from build123d import *

# Parameters (mm, degrees)
F0_W      = 200
F0_H      = 100
F1_DEPTH  = 20
F3_DEPTH  = 10
F5_DEPTH  = 10
F6_R      = 45
F7_DEPTH  = 10
F8_R      = 30
F9_DEPTH  = 32
F11_D     = 10
F11_DEPTH = 15
F11_TIP   = 3.0043030951


with BuildPart() as f1:
    # F0 (on Top) → F1 (new body)
    with BuildSketch(Plane.XY):
        Rectangle(F0_W, F0_H)
    extrude(amount=F1_DEPTH)

    # F2 (on face) → F3 (cut)
    with BuildSketch(Plane.XY.offset(20)):
        with BuildLine():
            Line((-75, 40), (-81, 40))
            ThreePointArc((-81, 40), (-89.4852813742, 36.4852813742), (-93, 28))
            Line((-93, 28), (-93, -28))
            ThreePointArc((-93, -28), (-89.4852813742, -36.4852813742), (-81, -40))
            Line((-81, -40), (-75, -40))
            ThreePointArc((-75, -40), (-66.5147186258, -36.4852813742), (-63, -28))
            Line((-63, -28), (-63, 28))
            ThreePointArc((-63, 28), (-66.5147186258, 36.4852813742), (-75, 40))
        make_face()
    extrude(amount=-F3_DEPTH, mode=Mode.SUBTRACT)

    # F4 (on face) → F5 (join)
    with BuildSketch(Plane.XY.offset(20)):
        with BuildLine():
            Line((45.028, 48), (-43, 48))
            ThreePointArc((-43, 48), (-50.0710678119, 45.0710678119), (-53, 38))
            Line((-53, 38), (-53, -38))
            ThreePointArc((-53, -38), (-50.0710678119, -45.0710678119), (-43, -48))
            Line((-43, -48), (45.028, -48))
            ThreePointArc((45.028, -48), (49.7542524478, -47.0300742427), (53.7164858981, -44.2770896333))
            Line((53.7164858981, -44.2770896333), (86.0406073726, -10.3463620417))
            ThreePointArc((86.0406073726, -10.3463620417), (90.18, 0), (86.0406073726, 10.3463620417))
            Line((86.0406073726, 10.3463620417), (53.7164858981, 44.2770896333))
            ThreePointArc((53.7164858981, 44.2770896333), (49.7542524478, 47.0300742427), (45.028, 48))
        make_face()
    extrude(amount=F5_DEPTH)

    # F6 (on face) → F7 (join)
    with BuildSketch(Plane.XY.offset(30)):
        Circle(F6_R)
    extrude(amount=F7_DEPTH)

    # F8 (on face) → F9 (cut)
    with BuildSketch(Plane.XY.offset(40)):
        Circle(F8_R)
    extrude(amount=-F9_DEPTH, mode=Mode.SUBTRACT)

    # F11
    with Locations(Plane.XY.offset(40)):
        with Locations((-37.5, 0), (0, 37.5), (37.5, 0), (0, -37.5)):
            Hole(F11_D / 2, depth=F11_DEPTH)
            with Locations((0, 0, -(F11_DEPTH + F11_TIP / 2))):  # 118° drill point
                Cone(0, F11_D / 2, F11_TIP, mode=Mode.SUBTRACT)


solid = f1.part
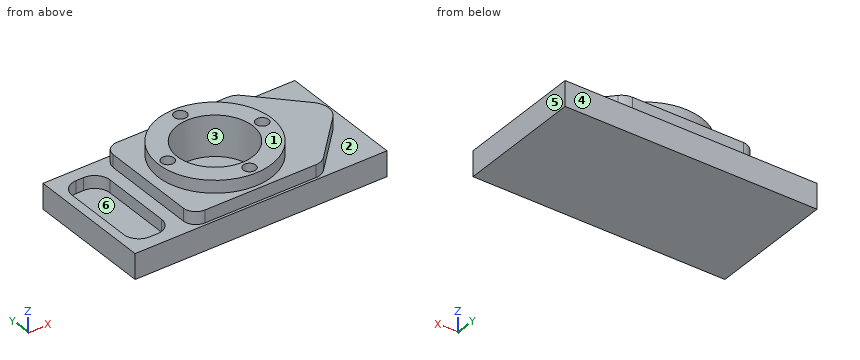
Model file for the job. Use its own axes, mm. Face numbers are marked on the shaded views. A direction names the side the tool comes from. Give positions to 0.01 mm unless a question says otherwise; leave off trailing zeros. Order: outer loops, then holes, each group sorted by start corner. A loop starts at its lowest first (then second) coordinate and runs counter-clockwise, first axis right, second up. Notation, with made-up numbers: (15, 34) - (32, 34) arc R26 ccw to (32, 50) - close; hole circle Ø1 at (-24, 28). An arc over 180 degrees is marked (long way). Write item = value, one per line. Start each with the question number.
1. Cut at A-A, the plane x = 14.5. List the corners of the cut face in (y, z).
2. Cut at D-D, the plane x = 50.5. List the corners of the cut face in (y, z), and give its area (3 significant figures).
3. Drop flat-ended pins along their axis: P1, Ø1, axis at y = 4.5, z = 21, coming from the +X side; P2, Ø3, axis at x = -1, z = 25, coming from the +Y side; P3, Ø9, axis at x = -85.5, y = 15.5, coming from the +Z side. Give the stop position or say it passes through.
4. Two-plate mould, pull along Y, no slides. Class the marked faces 3, 4, 5 and 6: pulls with the +Y half, pulls with the -Y half, needs draft (parallel to the pull), parting line crosses it, or undercut.
5. Probe line 1 along Y through (x, z) = (0, 29); line 2 along Z through (x, y) = (73, 35.5); line 3 along X through (y, z) = (-23, 18.5). List the from-to ranges inside material, lowest first.
6. Cut at B-B, the plane y = -26. List the corners of the cut face in (x, z).
7. Cut at C-C, the plane x = -21.5. List the corners of the cut face in (y, z).
8. Which spindle directions (+Z, -Z, +X, -X, +Y, -Y) get a long thin tool onto all of the face, cutting with end or side? Do the marked faces 1 and 2. Say none if no direction does.
Taken from the geometry:
q1.outline = (-50, 0) - (50, 0) - (50, 20) - (48, 20) - (48, 30) - (42.6, 30) - (42.6, 40) - (26.26, 40) - (26.26, 8) - (-26.26, 8) - (-26.26, 40) - (-42.6, 40) - (-42.6, 30) - (-48, 30) - (-48, 20) - (-50, 20) - close
q2.outline = (-50, 0) - (50, 0) - (50, 20) - (46.68, 20) - (46.68, 30) - (-46.68, 30) - (-46.68, 20) - (-50, 20) - close
q2.area = 2,930 mm²
q3.P1 = 89.64
q3.P2 = 48
q3.P3 = 10
q4.face_3 = undercut
q4.face_4 = pulls with the +Y half
q4.face_5 = needs draft
q4.face_6 = undercut
q5.line_1 = -48 to -42.5, -32.5 to -30, 30 to 32.5, 42.5 to 48
q5.line_2 = 0 to 20
q5.line_3 = -100 to -93, -63 to -19.26, 19.26 to 100
q6.outline = (-100, 0) - (100, 0) - (100, 20) - (71.13, 20) - (71.13, 30) - (36.73, 30) - (36.73, 40) - (14.97, 40) - (14.97, 8) - (-14.97, 8) - (-14.97, 40) - (-36.73, 40) - (-36.73, 30) - (-53, 30) - (-53, 20) - (-63, 20) - (-63, 10) - (-93, 10) - (-93, 20) - (-100, 20) - close
q7.outline = (-50, 0) - (50, 0) - (50, 20) - (48, 20) - (48, 30) - (39.53, 30) - (39.53, 40) - (20.92, 40) - (20.92, 8) - (-20.92, 8) - (-20.92, 40) - (-39.53, 40) - (-39.53, 30) - (-48, 30) - (-48, 20) - (-50, 20) - close
q8.face_1 = +Z, +X, -X, +Y, -Y
q8.face_2 = +Z
